Could you check a few things on this model? Use its own coordinates, in mm. Face numbers are marked on the shaded views. A direction names the side the tool comes from. Give positions to 0.01 mm unless a question says otherwise; leave off trailing zeros. Order: outer loops, then holes, each group sorted by start corner. A loop starts at its lowest first (then second) coordinate and runs counter-clockwise, first axis right, second up. Notation, with made-up numbers: (13.5, 25) - (42.5, 25) arc R15 ccw to (42.5, 40) - close; hole circle Ø4 at (7, 57.5). An arc over 180 degrees is marked (long way). Put each result on its own line as item: value.
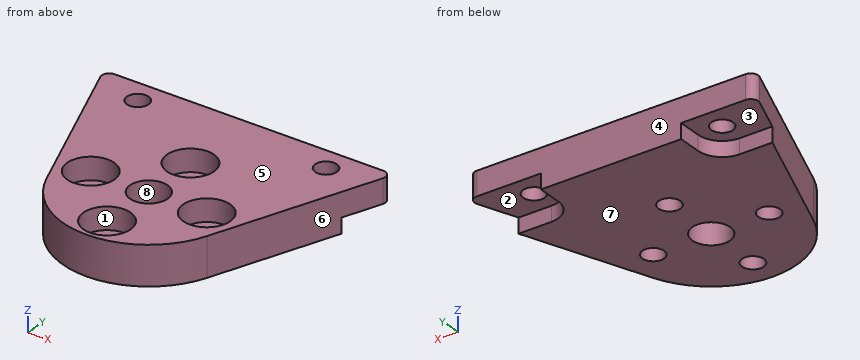
from build123d import *

# Parameters (mm, degrees)
SKETCH2_R                                           = 3.175
BOSS_EXTRUDE1_DEPTH                                 = 6.604
CBORE_FOR_6_BINDING_HEAD_MACHINE_SCREW1_D           = 3.6576
CBORE_FOR_6_BINDING_HEAD_MACHINE_SCREW1_CBORE_D     = 7.9375
CBORE_FOR_6_BINDING_HEAD_MACHINE_SCREW1_CBORE_DEPTH = 3.7338
F_6_CLEARANCE_HOLE1_D                               = 3.6576
CUT_EXTRUDE1_DEPTH                                  = 2.54
FILLET1_R                                           = 1.27


with BuildPart() as part:
    # Sketch2 → Boss-Extrude1 (new body)
    with BuildSketch(Plane.XY):
        with BuildLine():
            Line((24.4729, 18.9865), (13.523558965, -9.656158478))
            ThreePointArc((13.523558965, -9.656158478), (0, -18.964454722), (-13.523558965, -9.656158478))
            Line((-13.523558965, -9.656158478), (-24.4729, 18.9865))
            Line((-24.4729, 18.9865), (24.4729, 18.9865))
        make_face()
        with Locations(Location((0, -4.486454722, 0), (0, 0, 180))):
            Circle(SKETCH2_R, mode=Mode.SUBTRACT)
    extrude(amount=BOSS_EXTRUDE1_DEPTH)

    # CBORE for #6 Binding Head Machine Screw1 (through all)
    with Locations(Plane.XY.offset(6.604)):
        with Locations((0, -14.265454722), (0, 5.292545278), (9.779, -4.486454722), (-9.779, -4.486454722)):
            CounterBoreHole(CBORE_FOR_6_BINDING_HEAD_MACHINE_SCREW1_D / 2, CBORE_FOR_6_BINDING_HEAD_MACHINE_SCREW1_CBORE_D / 2, CBORE_FOR_6_BINDING_HEAD_MACHINE_SCREW1_CBORE_DEPTH)

    # #6 Clearance Hole1 (through all)
    with Locations(Plane(origin=(0, 0, 0), x_dir=(-1, 0, 0), z_dir=(0, 0, -1))):
        with Locations((15.875, 14.9987), (-15.875, 14.9987)):
            Hole(F_6_CLEARANCE_HOLE1_D / 2)

    # Sketch9 → Cut-Extrude1 (cut)
    with BuildSketch(Plane(origin=(0, 0, 0), x_dir=(-1, 0, 0), z_dir=(0, 0, -1))):
        with BuildLine():
            Line((-11.811, 14.9987), (-11.811, 18.9865))
            Line((-11.811, 18.9865), (-24.4729, 18.9865))
            Line((-24.4729, 18.9865), (-21.394906935, 10.9347))
            Line((-21.394906935, 10.9347), (-15.875, 10.9347))
            ThreePointArc((-15.875, 10.9347), (-13.001318041, 12.125018041), (-11.811, 14.9987))
        make_face()
        with BuildLine():
            Line((11.811, 14.9987), (11.811, 18.9865))
            Line((11.811, 18.9865), (24.4729, 18.9865))
            Line((24.4729, 18.9865), (21.394906935, 10.9347))
            Line((21.394906935, 10.9347), (15.875, 10.9347))
            ThreePointArc((15.875, 10.9347), (13.001318041, 12.125018041), (11.811, 14.9987))
        make_face()
    extrude(amount=-CUT_EXTRUDE1_DEPTH, mode=Mode.SUBTRACT)

    # Fillet1
    fillet1_edges = [part.edges().sort_by_distance(p)[0] for p in [
        (24.4729, 18.9865, 4.572),
        (-24.4729, 18.9865, 4.572),
    ]]
    fillet(fillet1_edges, radius=FILLET1_R)


solid = part.part
1) Suppose I cut it at A-A, the plane x = 0. List the corners of the cut face in (y, z) for me, and give its area (3 significant figures).
Filled in:
outline: (-18.96, 0) - (-16.09, 0) - (-16.09, 2.87) - (-18.23, 2.87) - (-18.23, 6.6) - (-18.96, 6.6) - close; (-12.44, 0) - (-7.66, 0) - (-7.66, 6.6) - (-10.3, 6.6) - (-10.3, 2.87) - (-12.44, 2.87) - close; (-1.31, 0) - (3.46, 0) - (3.46, 2.87) - (1.32, 2.87) - (1.32, 6.6) - (-1.31, 6.6) - close; (7.12, 0) - (18.99, 0) - (18.99, 6.6) - (9.26, 6.6) - (9.26, 2.87) - (7.12, 2.87) - close
area: 128 mm^2
2) We'd pull the mould along X, two halves only. Please class the marked faces 6, 7 and 8: pulls with the +X half, pulls with the -X half, needs draft (parallel to the pull), parting line crosses it, or undercut.
Filled in:
face 6: pulls with the +X half
face 7: needs draft
face 8: undercut
3) Suppose I cut it at C-C, the plane x = 17. List the corners of the cut face in (y, z) for me, and give its area (3 significant figures).
Filled in:
outline: (-0.56, 0) - (10.93, 0) - (10.93, 2.54) - (13.56, 2.54) - (13.56, 6.6) - (-0.56, 6.6) - close; (16.44, 2.54) - (18.99, 2.54) - (18.99, 6.6) - (16.44, 6.6) - close
area: 96.9 mm^2
4) Suppose I cut it at D-D, the plane z = 5.5. State how many separate pieces and enclosed holes the cut face has, and give its area (3 significant figures).
Filled in:
separate pieces: 1
enclosed holes: 7
area: 1,020 mm^2
5) I'm going to push flat-ended pins straight in: pin 1 (6 mm diameter, centred on x = 0, y = 5.29, fed in from +Z); pin 2 (3 mm diameter, centred on x = 15.88, y = 15, fed in from -Z); pin 3 (3 mm diameter, centred on y = 17, z = 1, fed in from +X); pin 4 (3 mm diameter, centred on y = -11, z = 5, fed in from -X). Where does each tip first touch, or does it pass through?
Filled in:
pin 1: stops at z = 2.87
pin 2: passes through
pin 3: stops at x = 11.81
pin 4: stops at x = -13.58
6) Which directions (+Z, -Z, +X, -X, +Y, -Y) give clear straight access to the entire face, cutting with the end or side of a thin tool? Please do the marked faces 1, 2, 3, 4 and 5.
Filled in:
face 1: +Z
face 2: -Z, +X, +Y
face 3: -Z, -X, +Y
face 4: +Z, -Z, +X, -X, +Y
face 5: +Z, +X, -X, +Y, -Y
7) If I drill on line 1 (Y direction, x = 0, z = 3.25); line 2 (Y direction, x = 0, z = 0.8); line 3 (X direction, y = 16, z = 4.25), over which ranges is the centre line in solid material (lowest first)? Write a range as [from, to].
Filled in:
line 1: y = [-18.96, -18.23], [-10.3, -7.66], [-1.31, 1.32], [9.26, 18.99]
line 2: y = [-18.96, -16.09], [-12.44, -7.66], [-1.31, 3.46], [7.12, 18.99]
line 3: x = [-23.33, -17.41], [-14.34, 14.34], [17.41, 23.33]
8) Suppose I cut it at B-B, the plane y = 14.5. List the corners of the cut face in (x, z) for me.
Filled in:
outline: (-22.76, 2.54) - (-17.63, 2.54) - (-17.63, 6.6) - (-22.76, 6.6) - close; (-14.12, 2.54) - (-11.84, 2.54) - (-11.84, 0) - (11.84, 0) - (11.84, 2.54) - (14.12, 2.54) - (14.12, 6.6) - (-14.12, 6.6) - close; (17.63, 2.54) - (22.76, 2.54) - (22.76, 6.6) - (17.63, 6.6) - close
